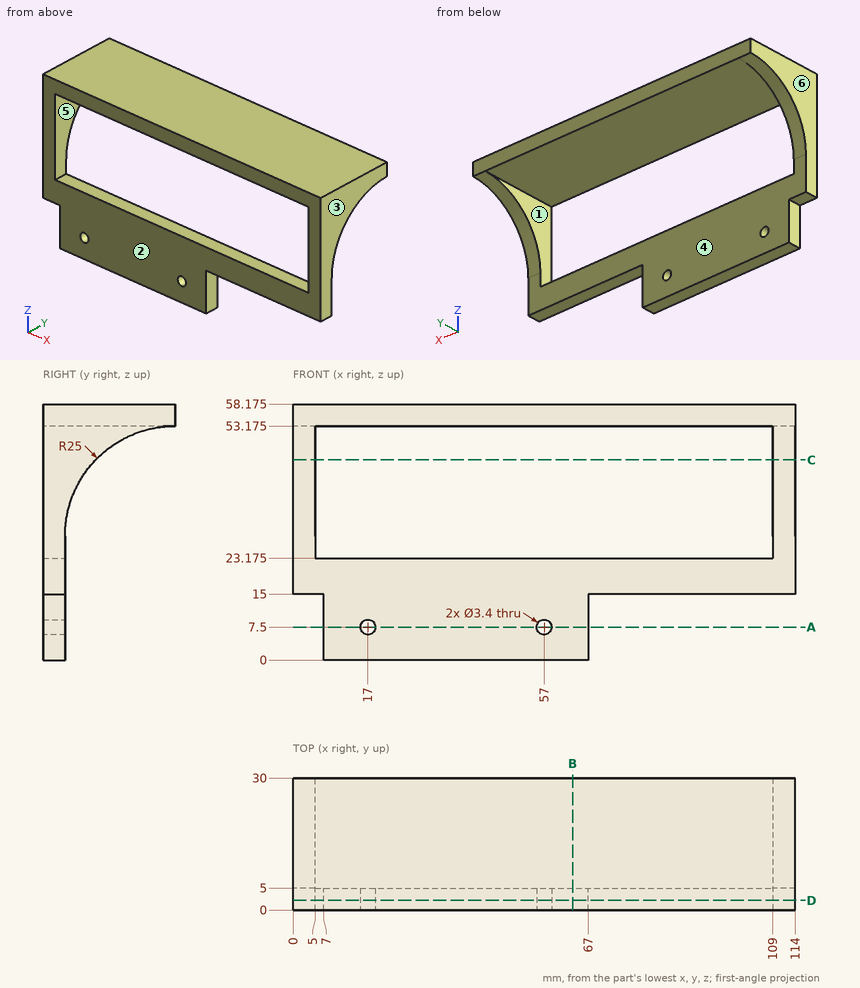
Drawing for the job (mm, zero at the part's lowest x, y, z). A direction names the side the tool comes from. Give positions to 0.01 mm unless a question says otherwise; leave off trailing zeros. Order: outer loops, then holes, each group sorted by start corner. A loop starts at its lowest first (then second) coordinate and runs counter-clockwise, first axis right, second up. Notation, with made-up numbers: M 45,63.5 L 82,63.5 A7 ccw 82,76.5 Z; hole C 30,-26 d4. An arc over 180 degrees is marked long. Write item = value, one per line. Start each with the question number.
(1) Slice it at B-B on x = 63.5. Write the cut outline in (y, z) (3 decimals), plus the area to 3 significant figures.
(2) Probe L1, parallel to X at y = 3.65, z = 7.5; L2, parallel to Z at x = 13, y = 2.75 (3 decimals); L3, parallel to X at y = 4.75, z = 50.5. List the from-to ranges inside material, lowest first. Write a range as [from, to].
(3) Slice it at C-C on z = 45.5. Write the cut outline in (x, y), plus the area to 3 significant figures.
(4) Which spindle directions (+Z, -Z, +X, -X, +Y, -Y) get a long thin tool onto all of the face, cutting with end or side? Do the marked faces 4, 5 and 6. Say none if no direction does.
(5) Slice it at A-A on z = 7.5. Write the cut outline in (x, y), plus the area to 3 significant figures.
(6) Slice it at D-D on y = 2.25. Write the cut outline in (x, z) (3 decimals), plus the area to 3 significant figures.
(7) Pin check, flat tips, straight feed: pin 1 Ø9 at (x, y) = (53, 17) entering from -Z (3 decimals); pin 2 Ø8.5 at (x, z) = (41, 8) entering from +Y; pin 3 Ø1.5 at (y, z) = (3, 9) entering from -X. Stop position of each tip, or through.
(8) Two-plate mould, pull along X, no slides. Class the marked faces 1, 2 and 3: released by +X, released by -X, zero draft, split by the parting line, or undercut.
Responses:
q1.outline = M 0,0 L 5,0 L 5,23.175 L 0,23.175 Z; M 0,53.175 L 30,53.175 L 30,58.175 L 0,58.175 Z
q1.area = 266 mm2
q2.L1 = [7, 15.3], [18.7, 55.3], [58.7, 67]
q2.L2 = [0, 23.175], [53.175, 58.175]
q2.L3 = [0, 5], [109, 114]
q3.outline = M 0,0 L 5,0 L 5,11.98 L 0,11.98 Z; M 109,0 L 114,0 L 114,11.98 L 109,11.98 Z
q3.area = 120 mm2
q4.face_4 = -Z, +X, -X, +Y
q4.face_5 = +Y, -Y
q4.face_6 = +Z, -Z, -X, +Y, -Y
q5.outline = M 7,0 L 15.3,0 L 15.3,5 L 7,5 Z; M 18.7,0 L 55.3,0 L 55.3,5 L 18.7,5 Z; M 58.7,0 L 67,0 L 67,5 L 58.7,5 Z
q5.area = 266 mm2
q6.outline = M 0,15 L 7,15 L 7,0 L 67,0 L 67,15 L 114,15 L 114,58.175 L 0,58.175 Z; hole M 5,23.175 L 109,23.175 L 109,53.175 L 5,53.175 Z; hole C 17,7.5 d3.4; hole C 57,7.5 d3.4
q6.area = 2,680 mm2
q7.pin_1 = 53.175
q7.pin_2 = 5
q7.pin_3 = 7
q8.face_1 = undercut
q8.face_2 = zero draft
q8.face_3 = released by +X
